Geometry: final body of the model. Coordinates: model frame, mm. A direction names the side the tool comes from. Round coordinates to 2 decimals unless told otherwise and drop trailing zeros. Write each loop counter-clockwise with the first axis right and the second up, starting at its lowest first coordinate (ties: lowest second). Pieces come first, ordered by that corner, then holes. Notation, with made-up numbers: (71, -16.5) - (106, -16.5) arc R36 cw to (106, 22.5) - close; hole circle Ø11 at (45, 34). An arc over 180 degrees is marked (long way). Write each question's results on one line, items separated by ' | '.
from build123d import *

# Parameters (mm, degrees)
SKETCH1_W           = 50.8
SKETCH1_H           = 25.4
SKETCH1_W_2         = 44.45
SKETCH1_H_2         = 19.05
BOSS_EXTRUDE1_DEPTH = 38.1
CUT_EXTRUDE1_REACH  = 54.363
SKETCH2_R           = 3.175
CUT_EXTRUDE2_REACH  = 54.363
SKETCH3_R           = 3.175


with BuildPart() as part:
    # Sketch1 → Boss-Extrude1 (new body)
    with BuildSketch(Plane(origin=(0, 0, 0), x_dir=(1, 0, 0), z_dir=(0, 1, 0))):
        Rectangle(SKETCH1_W, SKETCH1_H)
        Rectangle(SKETCH1_W_2, SKETCH1_H_2, mode=Mode.SUBTRACT)
    extrude(amount=BOSS_EXTRUDE1_DEPTH)

    # Sketch2 → Cut-Extrude1 (cut, up to next)
    with BuildSketch(Plane(origin=(0, 0, -12.7), x_dir=(-1, 0, 0), z_dir=(0, 0, -1)), mode=Mode.PRIVATE) as cut_extrude1_sk1:
        with Locations((0, 28.575)):
            Circle(SKETCH2_R)
    cut_extrude1_tool1 = extrude(cut_extrude1_sk1.sketch, amount=-CUT_EXTRUDE1_REACH, mode=Mode.PRIVATE) & part.part
    # Sketch2 → Cut-Extrude1 (cut, up to next)
    with BuildSketch(Plane(origin=(0, 0, -12.7), x_dir=(-1, 0, 0), z_dir=(0, 0, -1)), mode=Mode.PRIVATE) as cut_extrude1_sk2:
        with Locations((0, 9.525)):
            Circle(SKETCH2_R)
    cut_extrude1_tool2 = extrude(cut_extrude1_sk2.sketch, amount=-CUT_EXTRUDE1_REACH, mode=Mode.PRIVATE) & part.part
    add(cut_extrude1_tool1.solids().sort_by_distance((0, 28.575, -12.7))[0], mode=Mode.SUBTRACT)
    add(cut_extrude1_tool2.solids().sort_by_distance((0, 9.525, -12.7))[0], mode=Mode.SUBTRACT)

    # Sketch3 → Cut-Extrude2 (cut, up to next)
    with BuildSketch(Plane.XY.offset(12.7), mode=Mode.PRIVATE) as cut_extrude2_sk1:
        with Locations((15.875, 19.05)):
            Circle(SKETCH3_R)
    cut_extrude2_tool1 = extrude(cut_extrude2_sk1.sketch, amount=-CUT_EXTRUDE2_REACH, mode=Mode.PRIVATE) & part.part
    # Sketch3 → Cut-Extrude2 (cut, up to next)
    with BuildSketch(Plane.XY.offset(12.7), mode=Mode.PRIVATE) as cut_extrude2_sk2:
        with Locations((-15.875, 19.05)):
            Circle(SKETCH3_R)
    cut_extrude2_tool2 = extrude(cut_extrude2_sk2.sketch, amount=-CUT_EXTRUDE2_REACH, mode=Mode.PRIVATE) & part.part
    add(cut_extrude2_tool1.solids().sort_by_distance((15.875, 19.05, 12.7))[0], mode=Mode.SUBTRACT)
    add(cut_extrude2_tool2.solids().sort_by_distance((-15.875, 19.05, 12.7))[0], mode=Mode.SUBTRACT)


solid = part.part
Q1. Access query for faces 5 (the cylindrical face through (0.688, 25.476, -11.135)), 6 (the cylindrical face through (-14.41, 16.233, 11.135)), 7 (the flat face through (0, 19, 9.525)), 8 (the flat face through (25.4, 19, 0)). Directions: +Z, -Z, +X, -X, +Y, -Y. A direction counts if a zero-diameter tool reaches every point of the face in a straight line with its end or side. Return the directions, or none.
Answer block:
face 5: -Z | face 6: +Z | face 7: +Y, -Y | face 8: +Z, -Z, +X, +Y, -Y
Q2. Section query D-D, the plane x = 0. Return loops of the section in (y, z) (3 decimals), plus the area to 3 significant figures.
Answer block:
outline: (0, -12.7) - (6.35, -12.7) - (6.35, -9.525) - (0, -9.525) - close; (0, 9.525) - (38.1, 9.525) - (38.1, 12.7) - (0, 12.7) - close; (12.7, -12.7) - (25.4, -12.7) - (25.4, -9.525) - (12.7, -9.525) - close; (31.75, -12.7) - (38.1, -12.7) - (38.1, -9.525) - (31.75, -9.525) - close | area: 202 mm2
Q3. Section query A-A, the plane x = 8.5. Return loops of the section in (y, z) (3 decimals), plus the area to 3 significant figures.
Answer block:
outline: (0, -12.7) - (38.1, -12.7) - (38.1, -9.525) - (0, -9.525) - close; (0, 9.525) - (38.1, 9.525) - (38.1, 12.7) - (0, 12.7) - close | area: 242 mm2
Q4. Section query B-B, the plane z = -8. Return loops of the section in (x, y) (3 decimals), plus the area to 3 significant figures.
Answer block:
outline: (-25.4, 0) - (-22.225, 0) - (-22.225, 38.1) - (-25.4, 38.1) - close; (22.225, 0) - (25.4, 0) - (25.4, 38.1) - (22.225, 38.1) - close | area: 242 mm2
Q5. Mould query, pull axis Y, two halves, no side actions, for faces 1 (the flat face through (-25.4, 19, 0)), 2 (the cylindrical face through (17.34, 16.233, 11.135)), 3 (the cylindrical face through (-1.71, 12.2, -11.13)), 4 (the flat face through (0, 0, -10)). Classes: pulls with the +Y half, pulls with the -Y half, needs draft (parallel to the pull), parting line crosses it, or undercut.
Answer block:
face 1: needs draft | face 2: undercut | face 3: undercut | face 4: pulls with the -Y half
Q6. Ray query, line 1 along Y through (x, z) = (0, -11.1); line 2 along Z through (x, y) = (-17, 25) (3 decimals); line 3 along X through (y, z) = (33, -2.75) (3 decimals). Return the intervals inside material, ascending.
Answer block:
line 1: 0 to 6.35, 12.7 to 25.4, 31.75 to 38.1 | line 2: -12.7 to -9.525, 9.525 to 12.7 | line 3: -25.4 to -22.225, 22.225 to 25.4
Q7. Pin query (flat end, axial travel): pin 1 (5 mm diameter, centred on x = 0, y = 28.575, fed in from -Z) (3 decimals); pin 2 (6 mm diameter, centred on x = 9, z = 8, fed in from -Y). Return the tip coordinate at first contact, or that it passes through.
Answer block:
pin 1: z = 9.525 | pin 2: y = 0
Q8. Section query C-C, the plane y = 5. Return loops of the section in (x, z) (3 decimals).
Answer block:
outline: (-25.4, -12.7) - (25.4, -12.7) - (25.4, 12.7) - (-25.4, 12.7) - close; hole (-22.225, -9.525) - (22.225, -9.525) - (22.225, 9.525) - (-22.225, 9.525) - close
